CAD build for the part. Positions are in the model's coordinates, mm. Coordinates: 2 decimals unless noted, no trailing zeros. Put each result on its own line as item: value.
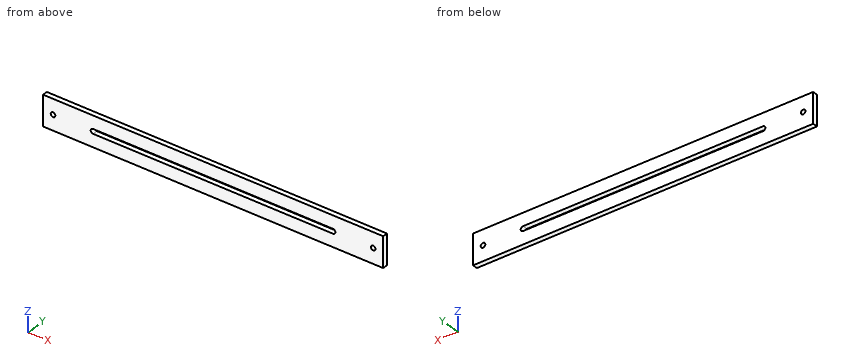
```python
from build123d import *

# Parameters (mm, degrees)
SKETCH1_W           = 215.9
SKETCH1_H           = 19.05
BOSS_EXTRUDE1_DEPTH = 3.175
SKETCH3_R           = 1.4605
CUT_EXTRUDE5_DEPTH  = 217.762065696


with BuildPart() as part:
    # Sketch1 → Boss-Extrude1 (new body)
    with BuildSketch(Plane(origin=(0, 0, 0), x_dir=(1, 0, 0), z_dir=(0, 1, 0))):
        with Locations((107.95, 9.525)):
            Rectangle(SKETCH1_W, SKETCH1_H)
    extrude(amount=BOSS_EXTRUDE1_DEPTH)

    # Sketch3 → Cut-Extrude5 (cut, through all)
    with BuildSketch(Plane(origin=(0, 3.175, 0), x_dir=(1, 0, 0), z_dir=(0, 1, 0))):
        with BuildLine():
            Line((184.15, 10.9855), (31.75, 10.9855))
            ThreePointArc((31.75, 10.9855), (30.2895, 9.525), (31.75, 8.0645))
            Line((31.75, 8.0645), (184.15, 8.0645))
            ThreePointArc((184.15, 8.0645), (185.6105, 9.525), (184.15, 10.9855))
        make_face()
        with Locations(Location((6.35, 9.525, 0), (0, 0, 270))):
            Circle(SKETCH3_R)
        with Locations(Location((209.55, 9.525, 0), (0, 0, 270))):
            Circle(SKETCH3_R)
    extrude(amount=-CUT_EXTRUDE5_DEPTH, mode=Mode.SUBTRACT)


solid = part.part
```
Q1. Pin check, flat tip, straight feed: pin 1 Ø4.5 at (x, z) = (209.55, -9.525) entering from -Y. Stop position of the tip, or through.
Determined:
pin 1: y = 0
Q2. Slice it at B-B, the plane y = 1.3. State how many separate pieces and enclosed holes the cut face has, then the cut area to 3 significant figures.
Determined:
separate pieces: 1
enclosed holes: 3
area: 3,650 mm2
Q3. Wall check: L1, parallel to Z at x = 134.5, y = 1.65. Give the ranges that are in metal, low to high. Write a range as from..to.
Determined:
L1: -19.05..-10.99, -8.06..0
